Could you check a few things on this model? Use its own coordinates, in mm. Face numbers are marked on the shaded views. A direction names the side the tool comes from. Coordinates: 2 decimals unless noted, no trailing zeros. Order: outer loops, then holes, each group sorted by start corner. A loop starts at its lowest first (then second) coordinate and runs counter-clockwise, first axis right, second up. Notation, with made-up numbers: (72, 29) - (83, 29) arc R23 ccw to (83, 60) - close; hole circle Ø7 at (64.5, -25.75). An arc over 180 degrees is marked (long way). Answer as a JSON object with one key per item and string values. Group by question number.
(1) Which directions (+Z, -Z, +X, -X, +Y, -Y) give clear straight access to the entire face, cutting with the end or side of a thin tool? Please do the marked faces 1 and 2.
(2) Will these pins go through, and if not, where does the flat tip stop? P1, Ø9.5, axis at x = 20, y = -50.5, coming from the +Z side; P2, Ø8, axis at x = -26, z = -16.5, coming from the -Y side; P3, Ø10, axis at x = 2.5, z = 2, coming from the -Y side; P4, Ø16, axis at y = -52, z = -3, coming from the +X side.
(3) Imagine slicing it at A-A, the plane y = -46.5. Write out the boundary of the cut face in (x, z), and give its area (3 significant figures).
(4) Imagine slicing it at C-C, the plane y = -22. Write out the boundary of the cut face in (x, z).
(5) Please list where these lines run through material, in increasing order: probe 1 along X at (y, z) = (-37.5, 8.5); probe 2 along Z at (x, y) = (11, -55); probe 3 along Y at (x, z) = (-4, -17.5).
(6) Imagine slicing it at B-B, the plane x = -20. Write out the boundary of the cut face in (y, z).
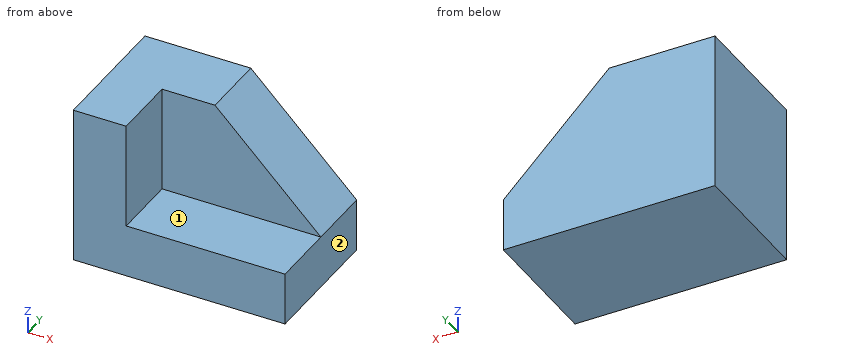
from build123d import *

# Parameters (mm, degrees)
F1_DEPTH = 63.5
F2_W     = 76.2
F2_H     = 31.75
F3_DEPTH = 50.8
F4_SIZE  = 50.8


with BuildPart() as f1:
    # F0 (on Front) → F1 (new body)
    with BuildSketch(Plane.XZ):
        Polygon((-29.114198, 20.572871), (-54.514198, 20.572871), (-54.514198, -55.627129), (47.085802, -55.627129), (47.085802, -30.227129), (-29.114198, -30.227129), align=None)
    extrude(amount=F1_DEPTH)

    # F2 (on face) → F3 (join)
    with BuildSketch(Plane.XY.offset(-30.227129)):
        with Locations((8.985802, -15.875)):
            Rectangle(F2_W, F2_H)
    extrude(amount=F3_DEPTH)

    # F4
    f4_edges = [f1.edges().sort_by_distance(p)[0] for p in [
        (47.085802, -15.875, 20.572871),
    ]]
    chamfer(f4_edges, length=F4_SIZE)


solid = f1.part
Result set:
{
 "1": {"face 1": "+Z, +X, -Y", "face 2": "+Z, -Z, +X, +Y, -Y"},
 "2": {"P1": "stops at z = -30.23", "P2": "stops at y = -63.5", "P3": "stops at y = -31.75", "P4": "stops at x = -29.11"},
 "3": {"outline": "(-54.51, -55.63) - (47.09, -55.63) - (47.09, -30.23) - (-29.11, -30.23) - (-29.11, 20.57) - (-54.51, 20.57) - close", "area": "3,870 mm^2"},
 "4": {"outline": "(-54.51, -55.63) - (47.09, -55.63) - (47.09, -30.23) - (-3.71, 20.57) - (-54.51, 20.57) - close"},
 "5": {"probe 1": "x = -54.51 to -29.11", "probe 2": "z = -55.63 to -30.23", "probe 3": "y = -31.75 to 0"},
 "6": {"outline": "(-63.5, -55.63) - (0, -55.63) - (0, 20.57) - (-31.75, 20.57) - (-31.75, -30.23) - (-63.5, -30.23) - close"}
}
